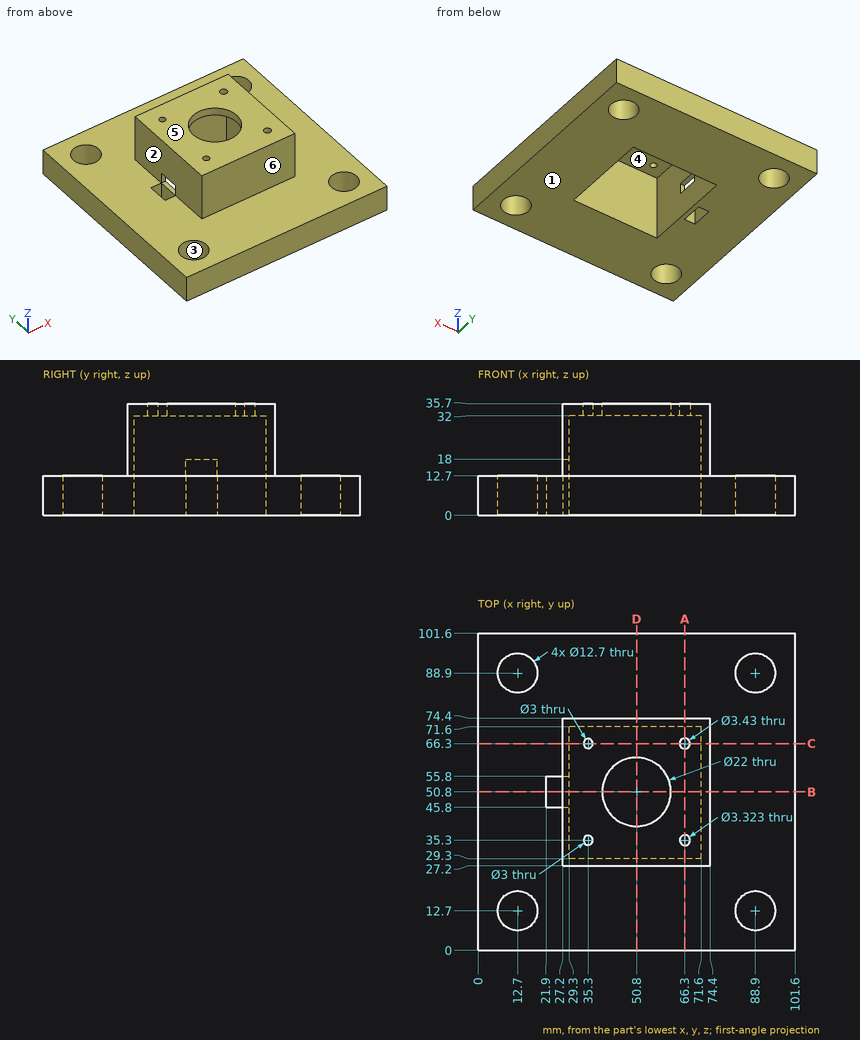
Source: three-view drawing plus pictorial views. Frame: mm from the lowest corner of the part. A direction names the side the tool comes from. Round coordinates to 2 decimals unless told otherwise and drop trailing zeros. Loops run counter-clockwise (first coordinate to the right, second up) from the corner with the lowest first, then second, coordinate; pieces in that order, holes last.
Q1. Pull-direction query (X, two-part tool) for the marked faces 1, 2 and 3; classes: released by +X, released by -X, zero draft, split by the parting line, or undercut.
Q2. Pin query (flat end, axial travel): P1, Ø1, axis at x = 89, y = 49.5, coming from the +Z side; P2, Ø2.5, axis at x = 66.3, y = 35.3, coming from the +Z side; P3, Ø18.5, axis at x = 57, z = 22, coming from the +Y side; P4, Ø1.7, axis at x = 28, z = 15, coming from the -Y side. Return the tip coordinate at first contact, or that it passes through.
Q3. Section C-C on y = 66.3. Return loops of the section in (x, z) (1 decimal).
Q4. Section B-B on y = 50.8. Return loops of the section in (x, z).
Q5. Material intervals for L1, parallel to Y at x = 35, z = 33; L2, parallel to Y at x = 12.7, z = 6.25; L3, parallel to Y at x = 50.8, z = 34.8, sorted ascending.
Q6. Access query for the marked faces 4, 5 and 6. Directions: +Z, -Z, +X, -X, +Y, -Y. A direction counts if a zero-diameter tool reaches every point of the face in a straight line with its end or side. Return the directions, or none.
Q7. Section A-A on x = 66.3. Return loops of the section in (y, z) (1 decimal).
Q8. Section D-D on x = 50.8. Return loops of the section in (y, z).
Evaluation:
1. face 1: zero draft
1. face 2: released by -X
1. face 3: undercut
2. P1: stops at z = 12.7
2. P2: passes through
2. P3: stops at y = 74.4
2. P4: stops at y = 27.2
3. outline: (0, 0) - (29.3, 0) - (29.3, 32) - (33.8, 32) - (33.8, 35.7) - (27.2, 35.7) - (27.2, 12.7) - (0, 12.7) - close; (36.8, 32) - (64.6, 32) - (64.6, 35.7) - (36.8, 35.7) - close; (68, 32) - (71.6, 32) - (71.6, 0) - (101.6, 0) - (101.6, 12.7) - (74.4, 12.7) - (74.4, 35.7) - (68, 35.7) - close
4. outline: (0, 0) - (21.9, 0) - (21.9, 12.7) - (0, 12.7) - close; (27.2, 0) - (29.3, 0) - (29.3, 12.7) - (27.2, 12.7) - close; (27.2, 18) - (29.3, 18) - (29.3, 32) - (39.8, 32) - (39.8, 35.7) - (27.2, 35.7) - close; (61.8, 32) - (71.6, 32) - (71.6, 0) - (101.6, 0) - (101.6, 12.7) - (74.4, 12.7) - (74.4, 35.7) - (61.8, 35.7) - close
5. L1: y = 27.2 to 33.83, 36.77 to 64.83, 67.77 to 74.4
5. L2: y = 0 to 6.35, 19.05 to 82.55, 95.25 to 101.6
5. L3: y = 27.2 to 39.8, 61.8 to 74.4
6. face 4: -Z
6. face 5: +Z, +X, -X, +Y, -Y
6. face 6: +Z, +X, -X, -Y
7. outline: (0, 0) - (29.3, 0) - (29.3, 32) - (33.6, 32) - (33.6, 35.7) - (27.2, 35.7) - (27.2, 12.7) - (0, 12.7) - close; (37, 32) - (64.6, 32) - (64.6, 35.7) - (37, 35.7) - close; (68, 32) - (71.6, 32) - (71.6, 0) - (101.6, 0) - (101.6, 12.7) - (74.4, 12.7) - (74.4, 35.7) - (68, 35.7) - close
8. outline: (0, 0) - (29.3, 0) - (29.3, 32) - (39.8, 32) - (39.8, 35.7) - (27.2, 35.7) - (27.2, 12.7) - (0, 12.7) - close; (61.8, 32) - (71.6, 32) - (71.6, 0) - (101.6, 0) - (101.6, 12.7) - (74.4, 12.7) - (74.4, 35.7) - (61.8, 35.7) - close
